Solid Edge part; units mm, degrees
sketch "Sketch1" plane through (0, 0, 0) normal (0, -1, 0) x (1, 0, 0)
  line L0 (-40, 0) -> (-70, 0)
  line L1 (0, -40) -> (0, -70)
  arc A0 (0, -40) -> (-40, 0) centre (0, 0) cw
  arc A1 (0, -70) -> (-70, 0) centre (0, 0) cw
extrude "Protrusion1" add sketch "Sketch1" along normal mid plane 30
sketch "Sketch2" plane through (0, 0, 0) normal (0, -1, 0) x (1, 0, 0)
  line L0 (23, -45) -> (23, -70)
  line L1 (23, -70) -> (-27, -70)
  line L2 (-27, -70) -> (-27, -45)
  line L3 (-27, -45) -> (23, -45)
revolve "RevolvedProtrusion_3" add sketch "Sketch2" angle 180 mid plane about axis through (-27, 0, -70) along (0, 0, 1)
sketch "Sketch3" plane through (0, 0, 0) normal (-1, 0, 0) x (0, -1, 0)
  line L0 (5, 0) -> (5, -24)
  line L1 (5, -24) -> (-5, -24)
  line L2 (-5, -24) -> (-5, 0)
  line L3 (-5, 0) -> (5, 0)
extrude "ExtrudedCutout_5" cut sketch "Sketch3" along normal blind 94.102
sketch "Sketch4" plane through (-2, 0, -45) normal (0, 0, 1) x (0, 1, 0)
  line L0 (-15, -7) -> (-15, -22.697)
  line L1 (0, -7) -> (-15, -7)
  line L2 (0, -7) -> (15, -7)
  line L3 (15, -7) -> (15, -22.697)
extrude "ExtrudedCutout_6" cut sketch "Sketch4" against normal blind 5 material side at (12.8485, -14.95, -45)
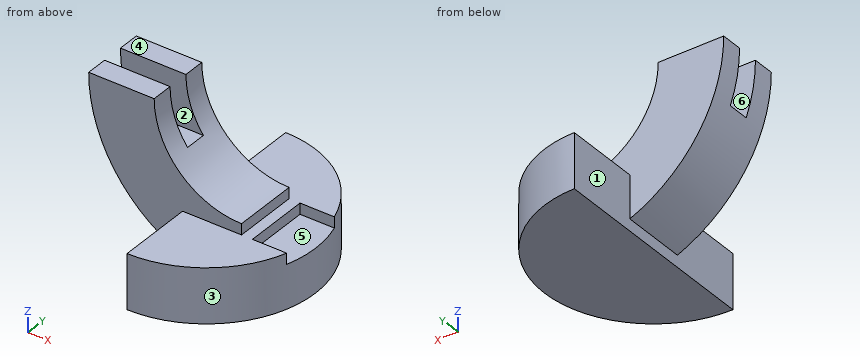
Build history of the part. All positions in model axes, mm. Face numbers are marked on the shaded views. A direction names the side the tool comes from. Round coordinates to 2 decimals unless told otherwise and drop trailing zeros. Order: outer loops, then holes, each group sorted by start corner. A loop starts at its lowest first (then second) coordinate and runs counter-clockwise, first axis right, second up. Notation, with made-up numbers: (-21.75, 31) - (-8.75, 31) arc R28 ccw to (-8.75, 60) - close; hole circle Ø5 at (-10, -36). An arc over 180 degrees is marked (long way). Use a Markdown table: item, result.
1) Pull direction Y, two halves, no side cores. Call the marked faces 1, 2 and 3: pulls with the +Y half, pulls with the -Y half, needs draft (parallel to the pull), parting line crosses it, or undercut.
Recorded:
| item | result |
|---|---|
| face 1 | needs draft |
| face 2 | undercut |
| face 3 | parting line crosses it |
2) Saw through at C-C on x = -6. Write the cut outline in (y, z), and give its area (3 significant figures).
Recorded:
| item | result |
|---|---|
| outline | (-45.38, -70) - (45.38, -70) - (45.38, -45) - (15, -45) - (15, -39.55) - (-15, -39.55) - (-15, -45) - (-45.38, -45) - close |
| area | 2,430 mm² |
3) Wall check: L1, parallel to Y at x = -43, z = -22; L2, parallel to Z at x = -24, y = -3; L3, parallel to Z at x = 9.5, y = 7. Give the ranges that are in metal, low to high.
Recorded:
| item | result |
|---|---|
| L1 | y = -15 to -5, 5 to 15 |
| L2 | z = -70 to -32 |
| L3 | z = -70 to -50 |
4) Saw through at B-B on y = 0. Write the cut outline in (x, z).
Recorded:
| item | result |
|---|---|
| outline | (-65.76, -24) arc R70 ccw to (-27, -64.58) - (-27, -70) - (23, -70) - (23, -50) - (5, -50) - (5, -45) - (0, -45) - (0, -40) arc R40 cw to (-32, -24) - close |
5) Saw through at A-A on z = -22. Write the cut outline in (x, y), and give its area (3 significant figures).
Recorded:
| item | result |
|---|---|
| outline | (-66.45, -15) - (-33.41, -15) - (-33.41, -5) - (-66.45, -5) - close; (-66.45, 5) - (-33.41, 5) - (-33.41, 15) - (-66.45, 15) - close |
| area | 661 mm² |
6) Flat gauge pins, fed straight in: pin 1 Ø3 at (x, y) = (-54, 1) entering from +Z; pin 2 Ø19.5 at (x, z) = (-23.5, -33) entering from -Y; pin 3 Ø6 at (x, z) = (-60.5, -20) entering from +Y; pin 4 Ø12 at (y, z) = (23.5, -13) entering from +X. Where does each tip first touch, or does it go through?
Recorded:
| item | result |
|---|---|
| pin 1 | stops at z = -24 |
| pin 2 | stops at y = -15 |
| pin 3 | stops at y = 15 |
| pin 4 | passes through |
7) Saw through at D-D on z = -63. Write the cut outline in (x, y), and give its area (3 significant figures).
Recorded:
| item | result |
|---|---|
| outline | (-30.51, -15) - (-27, -15) - (-27, -50) arc R50 ccw to (-27, 50) - (-27, 15) - (-30.51, 15) - close |
| area | 4,030 mm² |
8) Tool access for the marked faces 4, 5 and 6: list every direction of +Z, -Z, +X, -X, +Y, -Y with a clear straight run to the whole face (end or side of a thin tool).
Recorded:
| item | result |
|---|---|
| face 4 | +Z, +X, -X, +Y, -Y |
| face 5 | +Z, +X |
| face 6 | +Z, +X, -X |
